```python
from build123d import *

# Parameters (mm, degrees)
F0_R     = 6.35
F1_DEPTH = 25


with BuildPart() as f1:
    # F0 (on Top) → F1 (new body)
    with BuildSketch(Plane.XY):
        with BuildLine():
            ThreePointArc((60.325, 0), (58.139505, 6.07102), (52.585938, 9.35607))
            ThreePointArc((52.585938, 9.35607), (41.275, 0), (52.585938, -9.35607))
            ThreePointArc((52.585938, -9.35607), (58.139505, -6.07102), (60.325, 0))
        make_face()
        with Locations((50.8, 0)):
            Circle(F0_R, mode=Mode.SUBTRACT)
        with BuildLine():
            ThreePointArc((3.571875, 18.712141), (14.679011, 12.14204), (19.05, 0))
            ThreePointArc((19.05, 0), (14.679011, -12.14204), (3.571875, -18.712141))
            Line((3.571875, -18.712141), (52.585938, -9.35607))
            ThreePointArc((52.585938, -9.35607), (41.275, 0), (52.585938, 9.35607))
            Line((52.585938, 9.35607), (3.571875, 18.712141))
        make_face()
        with BuildLine():
            ThreePointArc((3.571875, -18.712141), (14.679011, -12.14204), (19.05, 0))
            ThreePointArc((19.05, 0), (14.679011, 12.14204), (3.571875, 18.712141))
            ThreePointArc((3.571875, 18.712141), (-19.05, 0), (3.571875, -18.712141))
        make_face()
        Circle(F0_R, mode=Mode.SUBTRACT)
    extrude(amount=F1_DEPTH)


solid = f1.part
```
CAD build for the part. Positions are in the model's coordinates, mm. Round coordinates to 2 decimals unless told otherwise and drop trailing zeros. Order: outer loops, then holes, each group sorted by start corner. A loop starts at its lowest first (then second) coordinate and runs counter-clockwise, first axis right, second up.
Q1. Slice it at A-A (x = 0). Write the cut outline in (y, z), and give its area (3 significant figures).
Q2. Drop flat-ended pins along their axis: pin 1 (6 mm diameter, centred on x = 44, z = 15, fed in from -Y); pin 2 (1 mm diameter, centred on y = 12, z = 4, fed in from -X); pin 3 (1.5 mm diameter, centred on y = 10.5, z = 6.5, fed in from -X). Give the stop position or say it passes through.
Q3. Wall check: L1, parallel to Y at x = 0, z = 7; L2, parallel to Y at x = 51.5, z = 16; L3, parallel to X at y = 6.5, z = 11.5. Give the ranges that are in metal, low to high.
Q4. Two-plate mould, pull along X, no slides. Class faces 1 (the cylindrical face through (-1.38, -6.2, 12.32)), 2 (the flat face through (11, 0, 25)), 3 (the flat face through (28.42, 13.97, 12.32)): pulls with the +X half, pulls with the -X half, needs draft (parallel to the pull), parting line crosses it, or undercut.
Q5. Slice it at B-B (z = 14.75). Write the cut outline in (x, y) (3 decimals), and give its area (3 significant figures).
Q6. Slice it at C-C (y = 4). Write the cut outline in (x, z).
Q7. Slice it at D-D (x = 50.8). Write the cut outline in (y, z).
Results below:
1. outline: (-19.05, 0) - (-6.35, 0) - (-6.35, 25) - (-19.05, 25) - close; (6.35, 0) - (19.05, 0) - (19.05, 25) - (6.35, 25) - close
1. area: 635 mm2
2. pin 1: stops at y = -11.57
2. pin 2: stops at x = -15.19
2. pin 3: stops at x = -16.37
3. L1: y = -19.05 to -6.35, 6.35 to 19.05
3. L2: y = -9.56 to -6.31, 6.31 to 9.56
3. L3: x = -17.91 to 57.76
4. face 1: undercut
4. face 2: needs draft
4. face 3: pulls with the +X half
5. outline: (3.572, -18.712) - (52.586, -9.356) arc R9.525 ccw to (60.325, 0) arc R9.525 ccw to (52.586, 9.356) - (3.572, 18.712) arc R19.05 ccw (long way) to start; hole circle Ø12.7 at (0, 0); hole circle Ø12.7 at (50.8, 0)
5. area: 1,940 mm2
6. outline: (-18.63, 0) - (-4.93, 0) - (-4.93, 25) - (-18.63, 25) - close; (4.93, 0) - (45.87, 0) - (45.87, 25) - (4.93, 25) - close; (55.73, 0) - (59.44, 0) - (59.44, 25) - (55.73, 25) - close
7. outline: (-9.7, 0) - (-6.35, 0) - (-6.35, 25) - (-9.7, 25) - close; (6.35, 0) - (9.7, 0) - (9.7, 25) - (6.35, 25) - close
